Source: CAD feature listing. Evaluate the final solid. Frame: model axes, mm. Face numbers are marked on the shaded views. A direction names the side the tool comes from. Round coordinates to 2 decimals unless told otherwise and drop trailing zeros. Order: outer loops, then holes, each group sorted by start corner. A loop starts at its lowest first (then second) coordinate and runs counter-clockwise, first axis right, second up. Notation, with made-up numbers: M -11,-25 L 37,-25 A11 ccw 37,-10 Z; hole C 80.25,51.5 d1. An arc over 180 degrees is marked long. Use one line per item in the form item = value. Start each with the question number.
Q1. Section A-A (z = 0). Return the cut outline in (x, y), plus the area to 3 significant figures.
Q2. Pull-direction query (Y, two-part tool) for the marked faces 5, 6 and 7; classes: pulls with the +Y half, pulls with the -Y half, needs draft (parallel to the pull), parting line crosses it, or undercut.
Q3. Section D-D (y = -3). Return the cut outline in (x, z).
Q4. Material intervals for probe 1 along Z at (x, y) = (16, 18.5); probe 2 along X at (y, z) = (-27, -34.5); probe 3 along Y at (x, z) = (12.5, -18), sorted ascending.
Q5. Section B-B (y = 17.5). Return the cut outline in (x, z), plus the area to 3 significant figures.
Q6. Section C-C (x = -11.5). Return the cut outline in (y, z), plus the area to 3 significant figures.
Q7. Contact query for flat-ended pins moving along their axis: pin 1 (4 mm diameter, centred on y = 15.5, z = 20.5, fed in from -X); pin 2 (2 mm diameter, centred on x = -27, y = -7, fed in from +Z); pin 3 (8 mm diameter, centred on x = 14, y = -20.5, fed in from +Z). Output: stop coordinate, or through.
Q8. Reachability of the marked faces 1, 2, 3 and 4 from +Z, -Z, +X, -X, +Y, -Y: full face, straight path, thin tool, end or side. Return the list, or none.
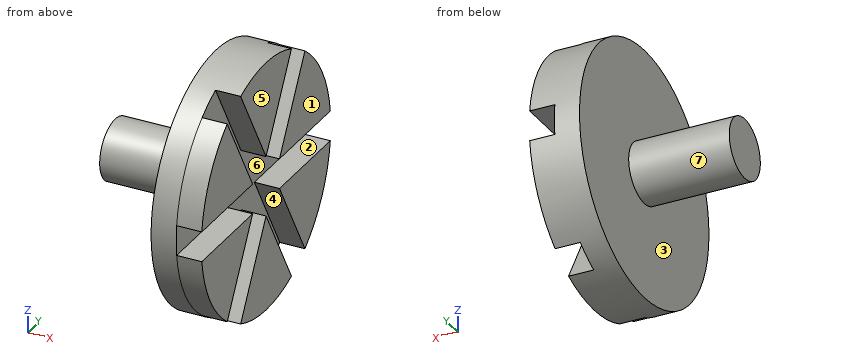
from build123d import *

# Parameters (mm, degrees)
SKETCH1_R           = 50
BOSS_EXTRUDE1_DEPTH = 10
BOSS_EXTRUDE2_DEPTH = 10
SKETCH9_R           = 12
BOSS_EXTRUDE3_DEPTH = 40


with BuildPart() as part:
    # Sketch1 → Boss-Extrude1 (new body)
    with BuildSketch(Plane(origin=(0, 0, 0), x_dir=(0, 0, -1), z_dir=(1, 0, 0))):
        Circle(SKETCH1_R)
    extrude(amount=BOSS_EXTRUDE1_DEPTH)

    # Sketch7 → Boss-Extrude2 (add)
    with BuildSketch(Plane(origin=(10, 0, 0), x_dir=(0, 0, -1), z_dir=(1, 0, 0))):
        with BuildLine():
            Line((12, 0), (45.98837052, -19.623194869))
            ThreePointArc((45.98837052, -19.623194869), (50, 0), (45.98837052, 19.623194869))
            Line((45.98837052, 19.623194869), (12, 0))
        make_face()
        with BuildLine():
            Line((6, -10.392304845), (6, -49.638694584))
            ThreePointArc((6, -49.638694584), (25, -43.301270189), (39.98837052, -30.015499715))
            Line((39.98837052, -30.015499715), (6, -10.392304845))
        make_face()
        with BuildLine():
            Line((6, 10.392304845), (39.98837052, 30.015499715))
            ThreePointArc((39.98837052, 30.015499715), (25, 43.301270189), (6, 49.638694584))
            Line((6, 49.638694584), (6, 10.392304845))
        make_face()
        with BuildLine():
            Line((-6, -10.392304845), (-39.98837052, -30.015499715))
            ThreePointArc((-39.98837052, -30.015499715), (-25, -43.301270189), (-6, -49.638694584))
            Line((-6, -49.638694584), (-6, -10.392304845))
        make_face()
        with BuildLine():
            Line((-12, 0), (-45.98837052, 19.623194869))
            ThreePointArc((-45.98837052, 19.623194869), (-50, 0), (-45.98837052, -19.623194869))
            Line((-45.98837052, -19.623194869), (-12, 0))
        make_face()
        with BuildLine():
            Line((-6, 10.392304845), (-6, 49.638694584))
            ThreePointArc((-6, 49.638694584), (-25, 43.301270189), (-39.98837052, 30.015499715))
            Line((-39.98837052, 30.015499715), (-6, 10.392304845))
        make_face()
    extrude(amount=BOSS_EXTRUDE2_DEPTH)

    # Sketch9 → Boss-Extrude3 (add)
    with BuildSketch(Plane.ZY):
        Circle(SKETCH9_R)
    extrude(amount=BOSS_EXTRUDE3_DEPTH)


solid = part.part
Results list:
q1.outline = M -40,-12 L 0,-12 L 0,-50 L 10,-50 L 10,50 L 0,50 L 0,12 L -40,12 Z
q1.area = 1,960 mm2
q2.face_5 = needs draft
q2.face_6 = undercut
q2.face_7 = parting line crosses it
q3.outline = M -40,-11.62 L 0,-11.62 L 0,-49.91 L 20,-49.91 L 20,-17.2 L 10,-17.2 L 10,17.2 L 20,17.2 L 20,49.91 L 0,49.91 L 0,11.62 L -40,11.62 Z
q4.probe_1 = -46.45 to -44.04, -20.04 to -6, 6 to 20.04, 44.04 to 46.45
q4.probe_2 = 0 to 20
q4.probe_3 = -46.65 to -17.32, -3.46 to 3.46, 17.32 to 46.65
q5.outline = M 0,-46.84 L 20,-46.84 L 20,-42.31 L 10,-42.31 L 10,-18.31 L 20,-18.31 L 20,-6 L 10,-6 L 10,6 L 20,6 L 20,18.31 L 10,18.31 L 10,42.31 L 20,42.31 L 20,46.84 L 0,46.84 Z
q5.area = 1,270 mm2
q6.outline = C 0,0 d24
q6.area = 452 mm2
q7.pin_1 = 0
q7.pin_2 = 10.39
q7.pin_3 = 47.2
q8.face_1 = +Z, -Z, +X, +Y, -Y
q8.face_2 = +X, +Y, -Y
q8.face_3 = -X
q8.face_4 = +X
